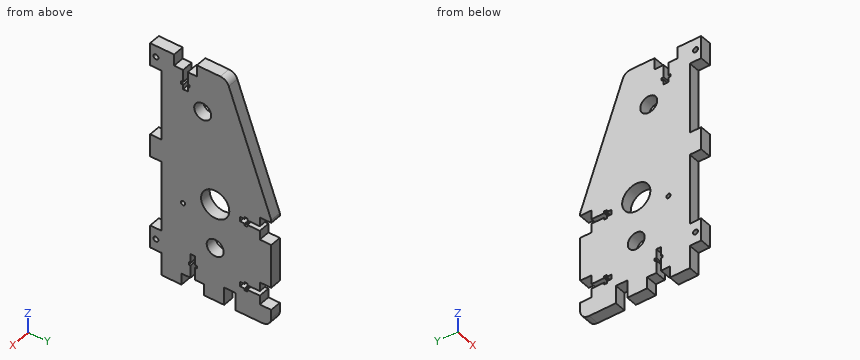
```python
from build123d import *

# Parameters (mm, degrees)
SKETCH2_R              = 1.4
BOSS_EXTRUDE1_DEPTH    = 6.35
SKETCH3_R              = 4.75
SKETCH3_R_2            = 7.9
AXII_DEPTH             = 76.241311791
CHAMFER1_SIZE          = 25
CHAMFER1_SIZE2         = 68.686935486
FILLET1_R              = 5
PLATEATTACHMENTS_DEPTH = 76.241311791
SKETCH6_R              = 1.2
WIREGUIDE_DEPTH        = 76.241311791


with BuildPart() as part:
    # Sketch2 → Boss-Extrude1 (new body)
    with BuildSketch(Plane(origin=(0, 0, 0), x_dir=(0, 0, -1), z_dir=(1, 0, 0))):
        Polygon((52.35, -30.7), (65.15, -30.7), (65.15, -19.55), (58.75, -19.55), (58.75, -14.5), (51.65, -14.5), (51.65, -15.5), (50.15, -15.5), (50.15, -14.5), (45.15, -14.5), (45.15, -11.9), (50.15, -11.9), (50.15, -10.9), (51.65, -10.9), (51.65, -11.9), (58.75, -11.9), (58.75, -6.85), (65.15, -6.85), (65.15, 4.3), (55.15, 4.3), (55.15, 10.7), (65.15, 10.7), (65.15, 30.7), (-65.15, 30.7), (-65.15, -30.7), (-65.15, -37.1), (-52.45, -37.1), (-52.45, -30.7), (-12.75, -30.7), (-12.75, -37.1), (-0.05, -37.1), (-0.05, -30.7), (39.65, -30.7), (39.65, -37.1), (52.35, -37.1), align=None)
        with Locations((-58.8, -33.9)):
            Circle(SKETCH2_R, mode=Mode.SUBTRACT)
        with Locations((46, -33.9)):
            Circle(SKETCH2_R, mode=Mode.SUBTRACT)
    extrude(amount=BOSS_EXTRUDE1_DEPTH)

    # Sketch3 → Axii (cut, through all)
    with BuildSketch(Plane(origin=(6.35, 0, 0), x_dir=(0, 0, -1), z_dir=(1, 0, 0))):
        with Locations((-40.15, -7.7)):
            Circle(SKETCH3_R)
        with Locations((34.85, -0.7)):
            Circle(SKETCH3_R)
        with Locations((9.85, -0.7)):
            Circle(SKETCH3_R_2)
    extrude(amount=-AXII_DEPTH, mode=Mode.SUBTRACT)

    # Chamfer1
    chamfer1_edges = [part.edges().sort_by_distance(p)[0] for p in [
        (3.175, 30.7, 65.15),
    ]]
    chamfer1_side = [part.faces().sort_by_distance(p)[0] for p in [
        (3.175, -3.2, 65.15),
    ]]
    chamfer(chamfer1_edges, length=CHAMFER1_SIZE, length2=CHAMFER1_SIZE2, reference=chamfer1_side[0])

    # Fillet1
    fillet1_edges = [part.edges().sort_by_distance(p)[0] for p in [
        (3.175, 5.7, 65.15),
        (3.175, 30.7, -65.15),
    ]]
    fillet(fillet1_edges, radius=FILLET1_R)

    # Sketch5 → PlateAttachments (cut, through all)
    with BuildSketch(Plane(origin=(6.35, 0, 0), x_dir=(0, 0, -1), z_dir=(1, 0, 0))):
        Polygon((55.15, 24.3), (55.15, 30.7), (42.45, 30.7), (42.45, 24.3), (47.5, 24.3), (47.5, 17.3), (46.4, 17.3), (46.4, 15.8), (47.5, 15.8), (47.5, 13.2), (50.1, 13.2), (50.1, 15.8), (51.2, 15.8), (51.2, 17.3), (50.1, 17.3), (50.1, 24.3), align=None)
        Polygon((17.85, 30.7), (5.15, 30.7), (5.15, 24.3), (10.2, 24.3), (10.2, 17.3), (9.1, 17.3), (9.1, 15.8), (10.2, 15.8), (10.2, 13.2), (12.8, 13.2), (12.8, 15.8), (13.9, 15.8), (13.9, 17.3), (12.8, 17.3), (12.8, 24.3), (17.85, 24.3), align=None)
        Polygon((-58.75, -11), (-65.15, -11), (-65.15, -23.7), (-58.75, -23.7), (-58.75, -18.65), (-51.75, -18.65), (-51.75, -19.75), (-50.25, -19.75), (-50.25, -18.65), (-47.65, -18.65), (-47.65, -16.05), (-50.25, -16.05), (-50.25, -14.95), (-51.75, -14.95), (-51.75, -16.05), (-58.75, -16.05), align=None)
    extrude(amount=-PLATEATTACHMENTS_DEPTH, mode=Mode.SUBTRACT)

    # Sketch6 → WireGuide (cut, through all)
    with BuildSketch(Plane(origin=(6.35, 0, 0), x_dir=(0, 0, -1), z_dir=(1, 0, 0))):
        with Locations((17.85, -18.7)):
            Circle(SKETCH6_R)
    extrude(amount=-WIREGUIDE_DEPTH, mode=Mode.SUBTRACT)


solid = part.part
```
Check sheet for the modelled part. Datum: model origin and axes. Units: mm. Give positions to 0.01 mm unless a question says otherwise; leave off trailing zeros. Write each loop counter-clockwise with the first axis right and the second up, starting at its lowest first coordinate (ties: lowest second). Pieces come first, ordered by that corner, then holes. Notation, with made-up numbers: (56.25, 46.25) - (99.25, 46.25) arc R6 ccw to (99.25, 51.25) - close; hole circle Ø7 at (76.25, 19.5). An arc over 180 degrees is marked (long way). Answer as a JSON object with one key per item and string values. Group by question number.
1) Sectioned sample at A-A (y = -33.9). Record the cut outline in (x, z), then the cut area to 3 significant figures.
2) Sectioned sample at C-C (x = 3.5). Give the number of separate pieces and of enclosed holes in the cut face, then the cut area to 3 significant figures.
3) Sectioned sample at D-D (z = 40.15). Record the cut outline in (x, y), then the cut area to 3 significant figures.
4) Thickness scan on probe 1 along Z at (x, y) = (4.25, -31); probe 2 along Y at (x, z) = (1.5, -10); probe 3 along Y at (x, z) = (2.25, -46). Record the ranges inside material, lowest first. Write a range as from..to.
5) Depth check by flat-ended pin: P1, Ø1.3, axis at x = 3, y = -13, coming from the -Z side; P2, Ø1.5, axis at x = 1.5, y = -14, coming from the +Z side; P3, Ø3, axis at x = 5, z = 23, coming from the +Y side. Enter the tip coordinate at first touch or a pass-through.
6) Sectioned sample at B-B (z = -34.85). Record the cut outline in (x, y).
Geometry results:
{
 "1": {"outline": "(0, -52.35) - (6.35, -52.35) - (6.35, -47.4) - (0, -47.4) - close; (0, -44.6) - (6.35, -44.6) - (6.35, -39.65) - (0, -39.65) - close; (0, 0.05) - (6.35, 0.05) - (6.35, 12.75) - (0, 12.75) - close; (0, 52.45) - (6.35, 52.45) - (6.35, 57.4) - (0, 57.4) - close; (0, 60.2) - (6.35, 60.2) - (6.35, 65.15) - (0, 65.15) - close", "area": "206 mm^2"},
 "2": {"separate pieces": "1", "enclosed holes": "6", "area": "6,500 mm^2"},
 "3": {"outline": "(0, -30.7) - (6.35, -30.7) - (6.35, -12.45) - (0, -12.45) - close; (0, -2.95) - (6.35, -2.95) - (6.35, 14.8) - (0, 14.8) - close", "area": "229 mm^2"},
 "4": {"probe 1": "z = -52.35..-39.65, 0.05..12.75, 52.45..65.15", "probe 2": "y = -30.7..-8.6, 7.2..15.8, 17.3..24.3", "probe 3": "y = -37.1..-35.3, -32.5..-14.5, -11.9..24.3"},
 "5": {"P1": "stops at z = -45.15", "P2": "stops at z = 58.75", "P3": "stops at y = 21.59"},
 "6": {"outline": "(0, -30.7) - (6.35, -30.7) - (6.35, -5.45) - (0, -5.45) - close; (0, 4.05) - (6.35, 4.05) - (6.35, 30.7) - (0, 30.7) - close"}
}
